from build123d import *

# Parameters (mm, degrees)
SKETCH1_W           = 75
SKETCH1_H           = 48
BOSS_EXTRUDE1_DEPTH = 3
SKETCH2_W           = 35
SKETCH2_H           = 22
CUT_EXTRUDE1_DEPTH  = 3
SKETCH3_W           = 75
SKETCH3_H           = 3
BOSS_EXTRUDE2_DEPTH = 33
SKETCH4_W           = 3
SKETCH4_H           = 42
BOSS_EXTRUDE3_DEPTH = 23
CUT_EXTRUDE2_DEPTH  = 70.276619433


with BuildPart() as part:
    # Sketch1 → Boss-Extrude1 (new body)
    with BuildSketch(Plane.XY):
        Rectangle(SKETCH1_W, SKETCH1_H)
    extrude(amount=BOSS_EXTRUDE1_DEPTH)

    # Sketch2 → Cut-Extrude1 (cut)
    with BuildSketch(Plane.XY.offset(3)):
        Rectangle(SKETCH2_W, SKETCH2_H)
    extrude(amount=-CUT_EXTRUDE1_DEPTH, mode=Mode.SUBTRACT)

    # Sketch3 → Boss-Extrude2 (add)
    with BuildSketch(Plane(origin=(0, 0, 0), x_dir=(-1, 0, 0), z_dir=(0, 0, -1))):
        with Locations((0, 22.5)):
            Rectangle(SKETCH3_W, SKETCH3_H)
        with Locations((0, -22.5)):
            Rectangle(SKETCH3_W, SKETCH3_H)
    extrude(amount=BOSS_EXTRUDE2_DEPTH)

    # Sketch4 → Boss-Extrude3 (add)
    with BuildSketch(Plane(origin=(0, 0, 0), x_dir=(-1, 0, 0), z_dir=(0, 0, -1))):
        with Locations((-36, 0)):
            Rectangle(SKETCH4_W, SKETCH4_H)
        with Locations((36, 0)):
            Rectangle(SKETCH4_W, SKETCH4_H)
    extrude(amount=BOSS_EXTRUDE3_DEPTH)

    # Sketch5 → Cut-Extrude2 (cut, through all)
    with BuildSketch(Plane.XZ.offset(24)):
        with BuildLine():
            Line((-30.5, -26), (30.5, -26))
            ThreePointArc((30.5, -26), (32.5, -28), (30.5, -30))
            Line((30.5, -30), (-30.5, -30))
            ThreePointArc((-30.5, -30), (-32.5, -28), (-30.5, -26))
        make_face()
    extrude(amount=-CUT_EXTRUDE2_DEPTH, mode=Mode.SUBTRACT)


solid = part.part
Design review of the part built by this model. Coordinates are the model's own, in mm. A direction names the side the tool comes from. Coordinates: 2 decimals unless noted, no trailing zeros. Loops run counter-clockwise (first coordinate to the right, second up) from the corner with the lowest first, then second, coordinate; pieces in that order, holes last. Notation, with made-up numbers: (-11, 53) - (47, 53) arc R14 cw to (47, 80) - close; hole circle Ø1 at (36, 63). An arc over 180 degrees is marked (long way). Use CSV: the item, a comma, the result in double quotes. Start each with the question number.
1. Mouldability with a two-part tool opening along X and no side actions: class faces 1 (the flat face through (-37.5, 0, -11)), 2 (the flat face through (0, -23, -30)), 3 (the flat face through (1, -22, -33)) as released by +X, released by -X, zero draft, split by the parting line, or undercut.
2. Add section C-C on x = 22.5. Give the boundary of the cut face in (y, z), plus the area to 3 significant figures.
3. Add section D-D on z = -16.5. Give the boundary of the cut face in (x, y), plus the area to 3 significant figures.
4. Add section A-A on z = -28. Give the boundary of the cut face in (x, y), plus the area to 3 significant figures.
5. Clearance check with flat-ended pins moving along their axes: pin 1 (0.9 mm diameter, centred on x = -36.5, y = 7, fed in from -Z); pin 2 (12.5 mm diameter, centred on x = 14.5, y = 8, fed in from -Z). State where each tip first meets the part, or that it passes through.
6. Add section B-B on y = 6. Give the boundary of the cut face in (x, z).
7. To check wall thickness, follow probe 1 along X at (y, z) = (-13, -16.5); probe 2 along Y at (x, z) = (26, -19.5); probe 3 along Z at (x, y) = (22.5, -0.5). State the ranges of each line that lie inside material, in increasing order.
8. For faces 4 (the cylindrical face through (-32.5, 22.5, -28)), 5 (the flat face through (36, 0, -23)), 6 (the flat face through (0, -11, 2)), 7 (the flat face through (1, -21, -16)), 8 (the flat face through (1, 24, -15)), list the 3-axis set-ups (+Z, -Z, +X, -X, +Y, -Y) from which the entire face can be reached by the end or side of a thin tool; tool diameter is ignored.
Resolved:
1,face 1,"released by -X"
1,face 2,"undercut"
1,face 3,"zero draft"
2,outline,"(-24, -33) - (-21, -33) - (-21, -30) - (-24, -30) - close; (-24, -26) - (-21, -26) - (-21, 0) - (21, 0) - (21, -26) - (24, -26) - (24, 3) - (-24, 3) - close; (21, -33) - (24, -33) - (24, -30) - (21, -30) - close"
2,area,"318 mm2"
3,outline,"(-37.5, -24) - (37.5, -24) - (37.5, 24) - (-37.5, 24) - close; hole (-34.5, -21) - (34.5, -21) - (34.5, 21) - (-34.5, 21) - close"
3,area,"702 mm2"
4,outline,"(-37.5, -24) - (-32.5, -24) - (-32.5, -21) - (-37.5, -21) - close; (-37.5, 21) - (-32.5, 21) - (-32.5, 24) - (-37.5, 24) - close; (32.5, -24) - (37.5, -24) - (37.5, -21) - (32.5, -21) - close; (32.5, 21) - (37.5, 21) - (37.5, 24) - (32.5, 24) - close"
4,area,"60.0 mm2"
5,pin 1,"z = -23"
5,pin 2,"z = 0"
6,outline,"(-37.5, -23) - (-34.5, -23) - (-34.5, 0) - (-17.5, 0) - (-17.5, 3) - (-37.5, 3) - close; (17.5, 0) - (34.5, 0) - (34.5, -23) - (37.5, -23) - (37.5, 3) - (17.5, 3) - close"
7,probe 1,"-37.5 to -34.5, 34.5 to 37.5"
7,probe 2,"-24 to -21, 21 to 24"
7,probe 3,"0 to 3"
8,face 4,"+Y, -Y"
8,face 5,"-Z, +X, -X"
8,face 6,"+Z, -Z"
8,face 7,"-Z"
8,face 8,"+Z, -Z, +X, -X, +Y"
